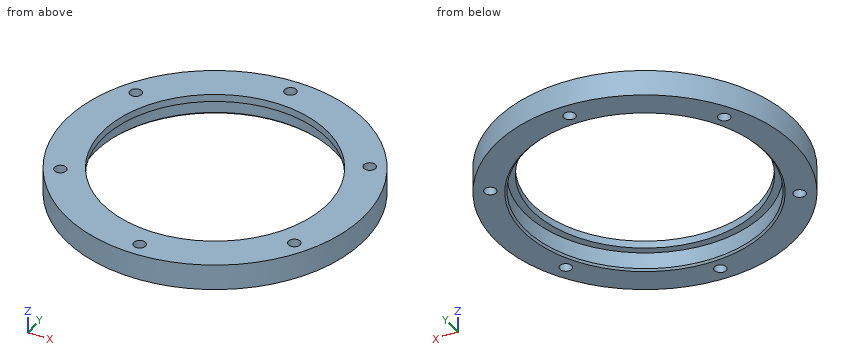
Autodesk Inventor part; units mm, degrees
ref_plane "YZ Plane" through (0, 0, 0) normal (1, 0, 0) x (0, 1, 0)
ref_plane "XZ Plane" through (0, 0, 0) normal (0, 1, 0) x (-1, 0, 0)
ref_plane "XY Plane" through (0, 0, 0) normal (0, 0, 1) x (1, 0, 0)
sketch "スケッチ1" plane through (0, 0, 0) normal (1, 0, 0) x (0, 1, 0)
  line L0 (32.6, 0) -> (32.6, 5)
  line L1 (32.6, 5) -> (30.6, 5)
  line L2 (30.6, 5) -> (30.6, 7)
  line L3 (30.6, 7) -> (40.6, 7)
  line L4 (40.6, 7) -> (40.6, 0)
  line L5 (40.6, 0) -> (32.6, 0)
  line L6 (0, -1.4) -> (0, 8.4)
  point P0 (0, 0)
  dimension "d0" = 32.6
  dimension "d1" = 5
  dimension "d2" = 2
  dimension "d3" = 2
  dimension "d22" = 8
revolve "回転1" add sketch "スケッチ1" angle 360 about axis through (0, 0, -10) along (0, 0, 1)
sketch "スケッチ2" plane through (0, 0, 7) normal (0, 0, 1) x (1, 0, 0)
  circle A0 centre (0, 0) radius 36.5
  point P0 (0, 36.5)
  point P1 (-31.6099, 18.25)
  point P2 (-31.6099, -18.25)
  point P3 (0, -36.5)
  point P4 (31.6099, -18.25)
  point P5 (31.6099, 18.25)
  dimension "d6" = 73
  dimension "d16" = 360
hole "穴1" at (31.6099, 18.25, 7) at (31.6099, -18.25, 7) at (0, -36.5, 7) at (-31.6099, -18.25, 7) at (-31.6099, 18.25, 7) at (0, 36.5, 7) direction (0, 0, -1) diameter 3.2 end through all
chamfer "面取り1" distance 0.5 angle 45 1 edges at (0, -32.6, 0)
properties part number "base2" material "ABS プラスチック"
Can you work these out from the model? Positions are in its coordinate system, mm. Give positions to 0.01 mm unless a question says otherwise; leave off trailing zeros. Order: outer loops, then holes, each group sorted by start corner. A loop starts at its lowest first (then second) coordinate and runs counter-clockwise, first axis right, second up. Notation, with made-up numbers: M 75,17.5 L 96,17.5 A18 ccw 96,21.5 Z; hole C -30,64 d5. An arc over 180 degrees is marked long. Write item = value, one per line. Start each with the question number.
Q1. I need wall thicknesses on probe 1 along Y at (x, z) = (0, 2.45); probe 2 along Y at (x, z) = (0, 5.7); probe 3 along X at (y, z) = (-18.25, 3.5). Which ranges of each line are inside material? Lowest first, please. Write a range as [from, to].
Q2. Suppose I cut it at B-B (z = 3.5). Write out the boundary of the cut face in (x, y), plus the area to 3 significant figures.
Q3. Suppose I cut it at D-D (y = 18.25). Count the separate pieces of the cut face and the enclosed holes in it, plus the area to 3 significant figures.
Q4. Will these pins go through, and if not, where does the flat tip stop? pin 1 Ø1.9 at (x, y) = (-31.61, 18.25) entering from -Z; pin 2 Ø1 at (y, z) = (16, 4.5) entering from -X; pin 3 Ø2 at (y, z) = (21, 4.5) entering from -X; pin 4 Ø1 at (y, z) = (-21, 3.5) entering from -X.
Q5. Suppose I cut it at C-C (y = -36.5). Write out the boundary of the cut face in (x, z), plus the area to 3 significant figures.
Q6. Suppose I cut it at A-A (y = 0). Write out the boundary of the cut face in (x, z).
Check result:
q1.probe_1 = [-40.6, -38.1], [-34.9, -32.6], [32.6, 34.9], [38.1, 40.6]
q1.probe_2 = [-40.6, -38.1], [-34.9, -30.6], [30.6, 34.9], [38.1, 40.6]
q1.probe_3 = [-36.27, -33.21], [-30.01, -27.01], [27.01, 30.01], [33.21, 36.27]
q2.outline = C 0,0 d81.2; hole C -31.61,-18.25 d3.2; hole C -31.61,18.25 d3.2; hole C 0,0 d65.2; hole C 0,-36.5 d3.2; hole C 0,36.5 d3.2; hole C 31.61,-18.25 d3.2; hole C 31.61,18.25 d3.2
q2.area = 1,790 mm2
q3.separate_pieces = 4
q3.enclosed_holes = 0
q3.area = 94.3 mm2
q4.pin_1 = through
q4.pin_2 = -37.52
q4.pin_3 = -35.33
q4.pin_4 = -35.04
q5.outline = M -17.78,0 L -1.6,0 L -1.6,7 L -17.78,7 Z; M 1.6,0 L 17.78,0 L 17.78,7 L 1.6,7 Z
q5.area = 227 mm2
q6.outline = M -40.6,0 L -33.1,0 L -32.6,0.5 L -32.6,5 L -30.6,5 L -30.6,7 L -40.6,7 Z; M 30.6,5 L 32.6,5 L 32.6,0.5 L 33.1,0 L 40.6,0 L 40.6,7 L 30.6,7 Z
